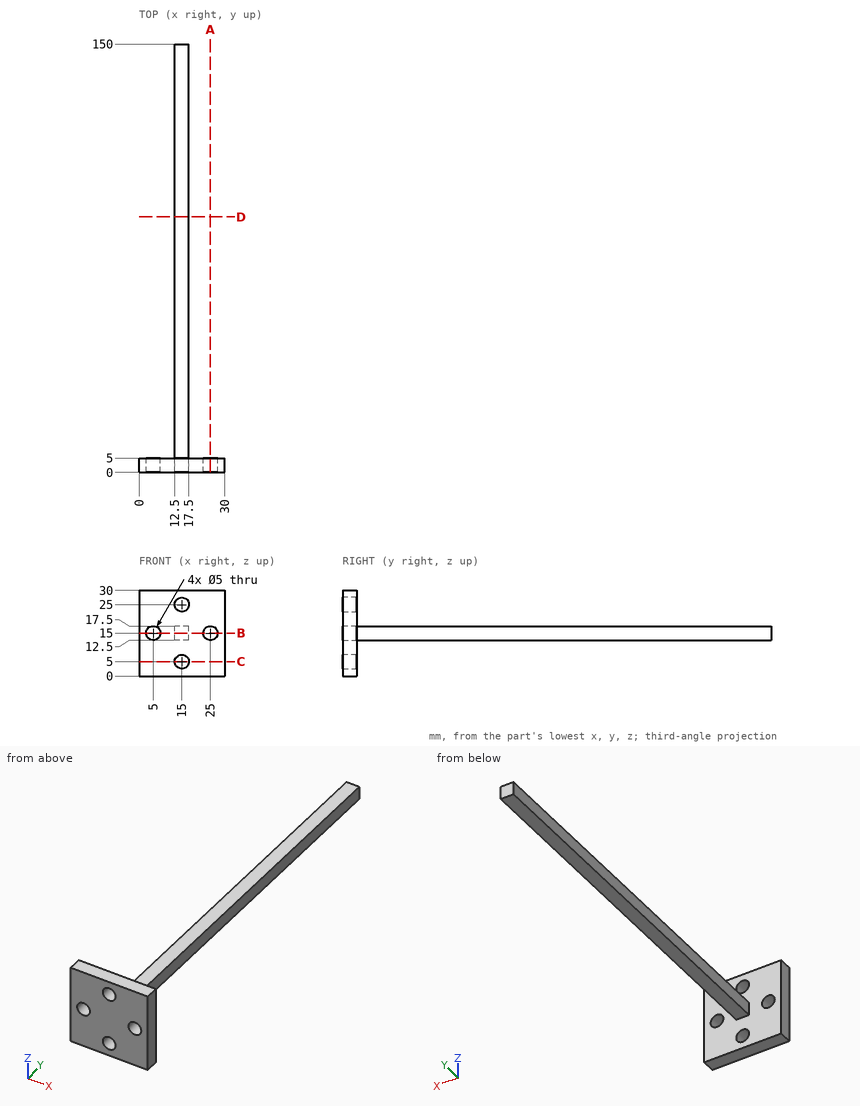
Design review of the part shown in the three views and the two pictorial views. Dimensions are in mm from the part's minimum x, y and z. Give positions to 0.01 mm unless a question says otherwise; leave off trailing zeros. Loops run counter-clockwise (first coordinate to the right, second up) from the corner with the lowest first, then second, coordinate; pieces in that order, holes last. Notation, with made-up numbers: (12, -2.75) - (62, -2.75) arc R21 cw to (62, 29.25) - close; hole circle Ø7 at (60, 20.5). An arc over 180 degrees is marked (long way). Answer as a JSON object with one key per item and string values.
Q1. Insertion check: pin 1 (5 mm diameter, centred on y = 112.5, z = 16, fed in from -X); pin 2 (5.5 mm diameter, centred on x = 14.5, y = 76, fed in from -Z); pin 3 (3 mm diameter, centred on x = 15, z = 25, fed in from -Y); pin 4 (12 mm diameter, centred on y = 30.5, z = 21.5, fed in from +X). Each pin has a flat end and moves straight along its axis. Give the tip position at first contact, or say it passes through.
Worked out:
{"pin 1": "stops at x = 12.5", "pin 2": "stops at z = 12.5", "pin 3": "passes through", "pin 4": "stops at x = 17.5"}
Q2. Add section A-A on x = 25. State the section outline as (y, z) points, plus the area to 3 significant figures.
Worked out:
{"outline": "(0, 0) - (5, 0) - (5, 12.5) - (0, 12.5) - close; (0, 17.5) - (5, 17.5) - (5, 30) - (0, 30) - close", "area": "125 mm^2"}
Q3. To check wall thickness, follow line 1 along X through (y, z) = (1.7, 15); line 2 along X through (y, z) = (3.4, 25); line 3 along Y through (x, z) = (11.5, 28). State the ranges of each line that lie inside material, in increasing order.
Worked out:
{"line 1": "x = 0 to 2.5, 7.5 to 22.5, 27.5 to 30", "line 2": "x = 0 to 12.5, 17.5 to 30", "line 3": "y = 0 to 5"}
Q4. Add section D-D on y = 89.5. State the section outline as (x, z) points.
Worked out:
{"outline": "(12.5, 12.5) - (17.5, 12.5) - (17.5, 17.5) - (12.5, 17.5) - close"}
Q5. Add section B-B on z = 15. State the section outline as (x, y) points, plus the area to 3 significant figures.
Worked out:
{"outline": "(0, 0) - (2.5, 0) - (2.5, 5) - (0, 5) - close; (7.5, 0) - (22.5, 0) - (22.5, 5) - (17.5, 5) - (17.5, 150) - (12.5, 150) - (12.5, 5) - (7.5, 5) - close; (27.5, 0) - (30, 0) - (30, 5) - (27.5, 5) - close", "area": "825 mm^2"}
Q6. Add section C-C on z = 5. State the section outline as (x, y) points, plus the area to 3 significant figures.
Worked out:
{"outline": "(0, 0) - (12.5, 0) - (12.5, 5) - (0, 5) - close; (17.5, 0) - (30, 0) - (30, 5) - (17.5, 5) - close", "area": "125 mm^2"}
